For this review, use the dimensioned drawing (mm, ordinates from the lowest corner) and the shaded views. A direction names the side the tool comes from. Coordinates: 2 decimals unless noted, no trailing zeros. Write each loop counter-clockwise with the first axis right and the second up, starting at its lowest first coordinate (ties: lowest second). Pieces come first, ordered by that corner, then holes. Notation, with made-up numbers: (-15.75, 13.25) - (43.25, 13.25) arc R22 cw to (43.25, 35.25) - close; hole circle Ø1 at (4.25, 48.5). An arc over 180 degrees is marked (long way). One line per item, written item: value.
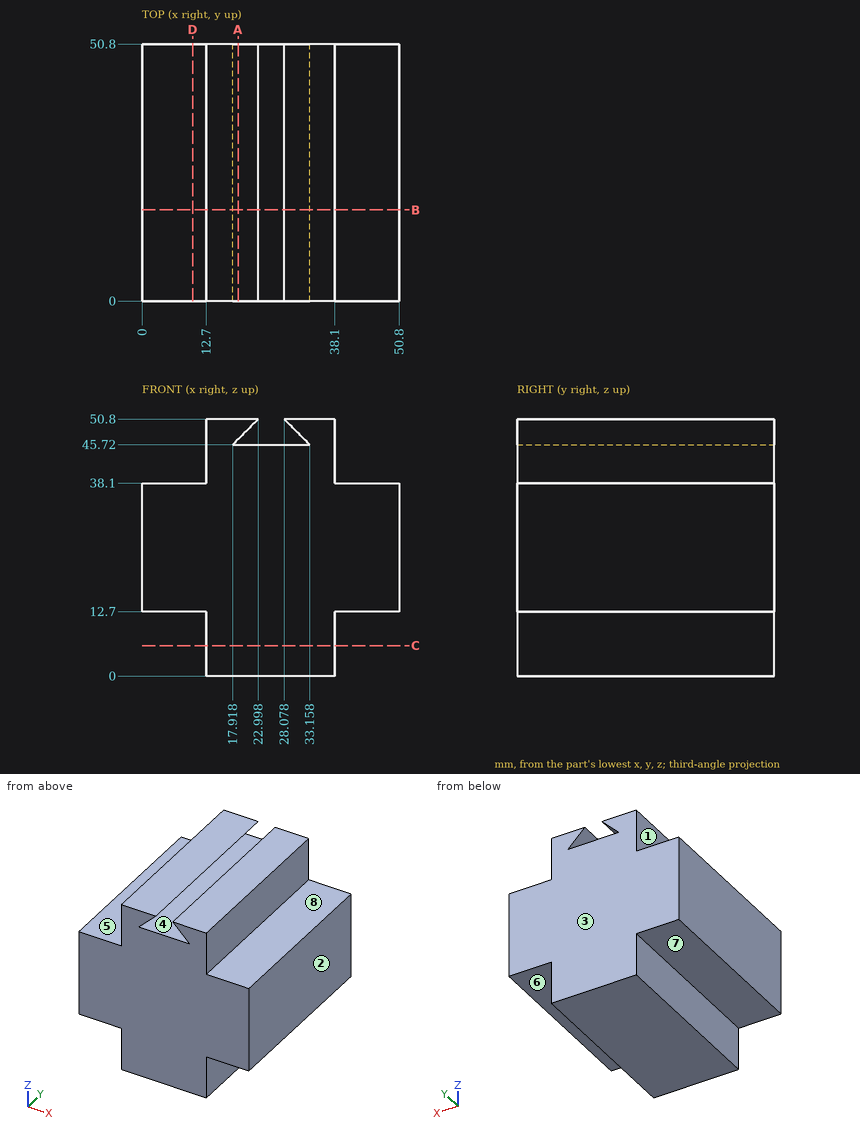
1. Insertion check: pin 1 Ø6.5 at (x, y) = (47, 32) entering from +Z; pin 2 Ø4 at (y, z) = (27.5, 9) entering from -X; pin 3 Ø6.5 at (x, y) = (42, 27) entering from -Z. Each pin has a flat end and moves straight along its axis. Give the tip position at first contact, or say it passes through.
Answer block:
pin 1: stops at z = 38.1
pin 2: stops at x = 12.7
pin 3: stops at z = 12.7
2. For the marked faces 5, 6, 7 and 8, list the 3-axis set-ups (+Z, -Z, +X, -X, +Y, -Y) from which the entire face can be reached by the end or side of a thin tool; tool diameter is ignored.
Answer block:
face 5: +Z, -X, +Y, -Y
face 6: -Z, +X, +Y, -Y
face 7: -Z, -X, +Y, -Y
face 8: +Z, +X, +Y, -Y
3. Wall thickness on line 1 along Z through (x, y) = (5, 32); line 2 along Z through (x, y) = (25.5, 10): over which ranges is each line inside the solid? List them lowest first.
Answer block:
line 1: z = 12.7 to 38.1
line 2: z = 0 to 45.72
4. Consider section D-D, the plane x = 10. Write out the cut boundary in (y, z), then the cut area to 3 significant figures.
Answer block:
outline: (0, 12.7) - (50.8, 12.7) - (50.8, 38.1) - (0, 38.1) - close
area: 1,290 mm^2
5. Mouldability with a two-part tool opening along X and no side actions: class the marked faces 1, 2, 3 and 4 as released by +X, released by -X, zero draft, split by the parting line, or undercut.
Answer block:
face 1: released by -X
face 2: released by +X
face 3: zero draft
face 4: undercut
6. Consider section B-B, the plane y = 18. Write out the cut boundary in (x, z).
Answer block:
outline: (0, 12.7) - (12.7, 12.7) - (12.7, 0) - (38.1, 0) - (38.1, 12.7) - (50.8, 12.7) - (50.8, 38.1) - (38.1, 38.1) - (38.1, 50.8) - (28.08, 50.8) - (33.16, 45.72) - (17.92, 45.72) - (23, 50.8) - (12.7, 50.8) - (12.7, 38.1) - (0, 38.1) - close
7. Consider section A-A, the plane x = 19. Write out the cut boundary in (y, z), then the cut area to 3 significant figures.
Answer block:
outline: (0, 0) - (50.8, 0) - (50.8, 45.72) - (0, 45.72) - close; (0, 46.8) - (50.8, 46.8) - (50.8, 50.8) - (0, 50.8) - close
area: 2,530 mm^2
8. Consider section C-C, the plane z = 6. Write out the cut boundary in (x, y).
Answer block:
outline: (12.7, 0) - (38.1, 0) - (38.1, 50.8) - (12.7, 50.8) - close
